The listing builds one solid part. Answer for the finished solid, in the listing's coordinates (mm). A direction names the side the tool comes from. Round coordinates to 2 decimals unless told otherwise and drop trailing zeros. Write each loop counter-clockwise with the first axis right and the second up, starting at its lowest first coordinate (ties: lowest second). Pieces come first, ordered by that corner, then holes. Notation, with made-up numbers: M 77,26 L 102,26 A21 ccw 102,53 Z; hole C 58,17 d9. An arc over 180 degrees is marked long. Write each question's results on one line, items separated by ' | '.
from build123d import *

# Parameters (mm, degrees)
SKETCH1_W                                      = 73
SKETCH1_H                                      = 40
BOSS_EXTRUDE1_DEPTH                            = 16
CUT_EXTRUDE1_DEPTH                             = 31
CUT_EXTRUDE2_REACH                             = 59.847
SKETCH14_R                                     = 6.5
CUT_EXTRUDE2_DIRECTION_2_REACH                 = 59.847
SKETCH15_R                                     = 1.595
CUT_EXTRUDE3_DEPTH                             = 4.32
SKETCH16_R                                     = 1.595
CUT_EXTRUDE4_DEPTH                             = 6.32
SKETCH18_R                                     = 1.595
CUT_EXTRUDE6_DEPTH                             = 6.32
SKETCH26_W                                     = 10
SKETCH26_H                                     = 40
BOSS_EXTRUDE2_DEPTH                            = 45
SKETCH27_R                                     = 1.595
CUT_EXTRUDE7_DEPTH                             = 97.509066932
SKETCH28_R                                     = 1.595
CUT_EXTRUDE10_DEPTH                            = 6.32
BOSS_EXTRUDE3_DEPTH                            = 1
SKETCH37_R                                     = 1.595
CUT_EXTRUDE14_DEPTH                            = 6.78
CUT_EXTRUDE15_START                            = -6.78
SKETCH38_R                                     = 1.595
CUT_EXTRUDE15_DEPTH                            = 6.78
SKETCH52_W                                     = 101.196897311
SKETCH52_H                                     = 58.467472524
CUT_EXTRUDE21_DEPTH                            = 9
CBORE_FOR_6_SOCKET_HEAD_CAP_SCREW1_D           = 3.7973
CBORE_FOR_6_SOCKET_HEAD_CAP_SCREW1_DEPTH       = 46.5
CBORE_FOR_6_SOCKET_HEAD_CAP_SCREW1_CBORE_D     = 9.68502
CBORE_FOR_6_SOCKET_HEAD_CAP_SCREW1_CBORE_DEPTH = 4.505198
CBORE_FOR_6_SOCKET_HEAD_CAP_SCREW1_TIP         = 1.140824014


# Read off the part's stored shape, not the designer's step: AdvancedHole3, AdvancedHole4
with BuildPart() as part:
    # Sketch1 → Boss-Extrude1 (new body)
    with BuildSketch(Plane(origin=(0, 0, 0), x_dir=(1, 0, 0), z_dir=(0, 1, 0))):
        Rectangle(SKETCH1_W, SKETCH1_H)
    extrude(amount=BOSS_EXTRUDE1_DEPTH)

    # Sketch5 → Cut-Extrude1 (cut)
    with BuildSketch(Plane(origin=(0, 0, -20), x_dir=(-1, 0, 0), z_dir=(0, 0, -1))):
        Polygon((17.965335593, 0), (24.220929062, 10.809975543), (36.5, 3.704235511), (36.5, 0), align=None)
    extrude(amount=-CUT_EXTRUDE1_DEPTH, mode=Mode.SUBTRACT)

    # Sketch14 → Cut-Extrude2 (cut, up to next)
    with BuildSketch(Plane(origin=(2.103927099, 16, -20), x_dir=(0, 0, 1), z_dir=(-0.8407935043817242, -0.5413559669842936, 0)), mode=Mode.PRIVATE) as cut_extrude2_sk1:
        with Locations(Location((15.40672826, 0.54117756, 0), (0, 0, 208.778472392))):
            Circle(SKETCH14_R)
    cut_extrude2_tool1 = extrude(cut_extrude2_sk1.sketch, amount=-CUT_EXTRUDE2_REACH, mode=Mode.PRIVATE) & part.part
    add(cut_extrude2_tool1.solids().sort_by_distance((1.810957, 16.455019, -4.593272))[0], mode=Mode.SUBTRACT)

    # Sketch14 → Cut-Extrude2 direction 2 (cut, up to next)
    with BuildSketch(Plane(origin=(2.103927099, 16, -20), x_dir=(0, 0, 1), z_dir=(-0.8407935043817242, -0.5413559669842936, 0)), mode=Mode.PRIVATE) as cut_extrude2_direction_2_sk1:
        with Locations(Location((15.40672826, 0.54117756, 0), (0, 0, 208.778472392))):
            Circle(SKETCH14_R)
    cut_extrude2_direction_2_tool1 = extrude(cut_extrude2_direction_2_sk1.sketch, amount=CUT_EXTRUDE2_DIRECTION_2_REACH, mode=Mode.PRIVATE) & part.part
    add(cut_extrude2_direction_2_tool1.solids().sort_by_distance((1.810957, 16.455019, -4.593272))[0], mode=Mode.SUBTRACT)

    # Sketch15 → Cut-Extrude3 (cut)
    with BuildSketch(Plane.ZY.offset(36.5)):
        with Locations((-14.800300311, 10.899842323)):
            Circle(SKETCH15_R)
        with Locations((5.199699689, 10.899842323)):
            Circle(SKETCH15_R)
    extrude(amount=-CUT_EXTRUDE3_DEPTH, mode=Mode.SUBTRACT)

    # Sketch16 → Cut-Extrude4 (cut)
    with BuildSketch(Plane(origin=(-13.45840239, -7.788203938, 0), x_dir=(0, 0, 1), z_dir=(-0.8655239452556988, -0.5008675475502585, 0))):
        with Locations(Location((-15.050029961, 13.487770019, 0), (0, 0, 270))):
            Circle(SKETCH16_R)
        with Locations(Location((4.949970039, 13.487770019, 0), (0, 0, 270))):
            Circle(SKETCH16_R)
    extrude(amount=-CUT_EXTRUDE4_DEPTH, mode=Mode.SUBTRACT)

    # Sketch18 → Cut-Extrude6 (cut)
    with BuildSketch(Plane.XY.offset(20)):
        with Locations((19, 8)):
            Circle(SKETCH18_R)
        with Locations((-19, 8)):
            Circle(SKETCH18_R)
    extrude(amount=-CUT_EXTRUDE6_DEPTH, mode=Mode.SUBTRACT)

    # Sketch26 → Boss-Extrude2 (add)
    with BuildSketch(Plane.XZ):
        with Locations((41.5, 0)):
            Rectangle(SKETCH26_W, SKETCH26_H)
    extrude(amount=-BOSS_EXTRUDE2_DEPTH)

    # Sketch27 → Cut-Extrude7 (cut, through all)
    with BuildSketch(Plane(origin=(46.5, 0, 0), x_dir=(0, 0, -1), z_dir=(1, 0, 0))):
        with Locations((5.05, 38.725)):
            Circle(SKETCH27_R)
        with Locations((13.298891971, 24.4375)):
            Circle(SKETCH27_R)
        with Locations((-3.198891971, 24.4375)):
            Circle(SKETCH27_R)
    extrude(amount=-CUT_EXTRUDE7_DEPTH, mode=Mode.SUBTRACT)

    # Sketch28 → Cut-Extrude10 (cut)
    with BuildSketch(Plane.XY.offset(20)):
        with Locations((41.5, 22.5)):
            Circle(SKETCH28_R)
    extrude(amount=-CUT_EXTRUDE10_DEPTH, mode=Mode.SUBTRACT)

    # Sketch33 → Boss-Extrude3 (add)
    with BuildSketch(Plane(origin=(0, 0, -20), x_dir=(-1, 0, 0), z_dir=(0, 0, -1))):
        Polygon((-46.5, 45), (-36.5, 45), (-36.5, 16), (36.5, 16), (36.5, 3.704235511), (24.220929062, 10.809975543), (17.965335593, 0), (-46.5, 0), align=None)
    extrude(amount=BOSS_EXTRUDE3_DEPTH)

    # Sketch37 → Cut-Extrude14 (cut)
    with BuildSketch(Plane.ZY.offset(36.5)):
        with Locations((15.5, 7.999173791)):
            Circle(SKETCH37_R)
    extrude(amount=-CUT_EXTRUDE14_DEPTH, mode=Mode.SUBTRACT)

    # Sketch38 → Cut-Extrude15 (cut)
    with BuildSketch(Plane(origin=(46.5, 0, 0), x_dir=(0, 0, -1), z_dir=(1, 0, 0)).offset(CUT_EXTRUDE15_START)):
        with Locations(Location((-15.5, 7.999173791, 0), (0, 0, 180))):
            Circle(SKETCH38_R)
    extrude(amount=CUT_EXTRUDE15_DEPTH, mode=Mode.SUBTRACT)

    # Sketch52 → Cut-Extrude21 (cut)
    with BuildSketch(Plane(origin=(0, 0, 11), x_dir=(-1, 0, 0), z_dir=(0, 0, -1))):
        with Locations((-4.130814665, 20.01964795)):
            Rectangle(SKETCH52_W, SKETCH52_H)
    extrude(amount=-CUT_EXTRUDE21_DEPTH, mode=Mode.SUBTRACT)

    # CBORE for #6 Socket Head Cap Screw1
    with Locations(Plane(origin=(46.5, 0, 0), x_dir=(0, 0, -1), z_dir=(1, 0, 0))):
        with Locations((5.05, 38.725), (13.298891971, 24.4375), (-3.198891971, 24.4375)):
            CounterBoreHole(CBORE_FOR_6_SOCKET_HEAD_CAP_SCREW1_D / 2, CBORE_FOR_6_SOCKET_HEAD_CAP_SCREW1_CBORE_D / 2, CBORE_FOR_6_SOCKET_HEAD_CAP_SCREW1_CBORE_DEPTH, depth=CBORE_FOR_6_SOCKET_HEAD_CAP_SCREW1_DEPTH)
            with Locations((0, 0, -(CBORE_FOR_6_SOCKET_HEAD_CAP_SCREW1_DEPTH + CBORE_FOR_6_SOCKET_HEAD_CAP_SCREW1_TIP / 2))):  # 118° drill point
                Cone(0, CBORE_FOR_6_SOCKET_HEAD_CAP_SCREW1_D / 2, CBORE_FOR_6_SOCKET_HEAD_CAP_SCREW1_TIP, mode=Mode.SUBTRACT)

    # AdvancedHole3 outline → AdvancedHole3 (revolve, cut)
    with BuildSketch(Plane(origin=(-1.5, 8, 0), x_dir=(1, 0, 0), z_dir=(0, -1, 0))):
        Polygon((0.889, -21), (0.889, -17.000000126), (0, -16.465835036), (0, -21), align=None)
    revolve(axis=Axis((-1.5, 8, 0), (0, 0, 1)), mode=Mode.SUBTRACT)

    # AdvancedHole3 2 outline → AdvancedHole3 2 (revolve, cut)
    with BuildSketch(Plane(origin=(31.5, 8, 0), x_dir=(1, 0, 0), z_dir=(0, -1, 0))):
        Polygon((0.889, -21), (0.889, -17.000000126), (0, -16.465835036), (0, -21), align=None)
    revolve(axis=Axis((31.5, 8, 0), (0, 0, 1)), mode=Mode.SUBTRACT)

    # AdvancedHole4 outline → AdvancedHole4 (revolve, cut)
    with BuildSketch(Plane(origin=(-1.5, 8, 0), x_dir=(1, 0, 0), z_dir=(0, -1, 0))):
        Polygon((0, 6.465835036), (0.889, 7.000000126), (0.889, 11), (0, 11), align=None)
    revolve(axis=Axis((-1.5, 8, 0), (0, 0, 1)), mode=Mode.SUBTRACT)

    # AdvancedHole4 2 outline → AdvancedHole4 2 (revolve, cut)
    with BuildSketch(Plane(origin=(31.5, 8, 0), x_dir=(1, 0, 0), z_dir=(0, -1, 0))):
        Polygon((0, 6.465835036), (0.889, 7.000000126), (0.889, 11), (0, 11), align=None)
    revolve(axis=Axis((31.5, 8, 0), (0, 0, 1)), mode=Mode.SUBTRACT)


solid = part.part
1) A tool of negligible diameter and unlimited length cuts with its end or side. For faces 1 (the face through (-14.755, 7.071, -15.028)), 2 (the face through (-30.446, 7.207, -4.776)), 3 (the face through (36.5, 31, -5)), 4 (the face through (-1.69, 7.13, 9.03)), 5 (the face through (41.995, 38.8, -7.1)), from which of +Z, -Z, +X, -X, +Y, -Y can it reach the whole face along a straight path? Write none if from no direction.
Return value:
face 1: none | face 2: +Z, -Z, -Y | face 3: +Z, -Z, -X, +Y | face 4: +Z | face 5: +X
2) Section B-B (y = 28) is taken. Determine the outline of the cut face in (x, z).
Return value:
outline: M 36.5,-21 L 46.5,-21 L 46.5,-16.58 L 41.99,-16.58 L 41.99,-10.02 L 46.5,-10.02 L 46.5,-0.08 L 41.99,-0.08 L 41.99,6.48 L 46.5,6.48 L 46.5,11 L 36.5,11 Z
3) The mould has two halves that part along Z. Classify faces 6 (the face through (-1.52, 8.153, 6.559)), 7 (the face through (-17.69, 5.746, -16.607)), 8 (the face through (-1.69, 7.13, -18.97)): +Z half, -Z half, draft (parallel to the pull), parting line (faces both ways), or undercut.
Return value:
face 6: +Z half | face 7: undercut | face 8: draft
4) Section A-A (z = -5.05) is taken. Determine the outline of the cut face in (x, y).
Return value:
outline: M -36.5,3.7 L -24.22,10.81 L -22.79,8.33 L -10.87,16 L -36.5,16 Z; M -11.77,0 L 46.5,0 L 46.5,33.88 L 41.99,33.88 L 41.99,36.83 L 36.5,36.83 L 36.5,16 L 13.08,16 Z; M 36.5,40.62 L 41.99,40.62 L 41.99,43.57 L 46.5,43.57 L 46.5,45 L 36.5,45 Z
5) Find the intervals of material crossed by line 1 (Y direction, x = 39, z = -5); line 2 (Y direction, x = 8.5, z = -19); line 3 (X direction, y = 9.5, z = -8), in increasing order.
Return value:
line 1: 0 to 36.83, 40.62 to 45 | line 2: 0 to 16 | line 3: -36.5 to -26.48, -23.46 to -19.22, 1.23 to 46.5
6) Each of these flat-tipped pins is pushed along its axis until it touches: pin 1 (5 mm diameter, centred on y = 23.5, z = -12.5, fed in from +X); pin 2 (8.5 mm diameter, centred on y = 24.44, z = 3.2, fed in from -X); pin 3 (10 mm diameter, centred on x = 33.5, z = -5.5, fed in from +Y); pin 4 (1.1 mm diameter, centred on x = -1.5, y = 8, fed in from -Z). Where does it stop, or does it pass through?
Return value:
pin 1: x = 41.99 | pin 2: x = 36.5 | pin 3: y = 45 | pin 4: z = -16.8
